Check sheet for the modelled part. Datum: model origin and axes. Units: mm. Coordinates: 2 decimals unless noted, no trailing zeros. Write each loop counter-clockwise with the first axis right and the second up, starting at its lowest first coordinate (ties: lowest second). Pieces come first, ordered by that corner, then holes. Notation, with made-up numbers: (60, -10) -> (74, -10) arc R20 cw to (74, 6) -> close; hole circle Ø2 at (-14.75, 35). An arc over 180 degrees is marked (long way). One line per item, written item: value. Start each with the question number.
1) Sectioned sample at C-C on z = -468.5. Enter the section's corners in (x, y) (3 decimals).
2) Scan lines: line 1 along Z through (x, y) = (0.95, 40.5); line 2 along Z through (x, y) = (2.95, 4.5); line 3 along Z through (x, y) = (0.9, 41). Record each from-to range of solid material in increasing order. Write a range as [from, to].
3) Sectioned sample at A-A on z = -557.53. Enter the section's corners in (x, y) (3 decimals), plus the area to 3 significant figures.
4) Gauge pin test, flat ends, axial feed: P1, Ø5.5, axis at y = 15.875, z = -431.8, coming from the +X side; P2, Ø1.6, axis at x = 1, z = -849, coming from the +Y side; P3, Ø1.5, axis at x = 2, z = -437, coming from the -Y side (3 decimals); P4, Ø1, axis at x = 1.5, y = 59, coming from the +Z side. Record the tip position at first contact, or that the pin passes through.
5) Sectioned sample at B-B on x = 2.6. Give the number of separate pieces and of enclosed holes in the cut face, plus the area to 3 significant figures.
Autodesk Inventor part; units mm, degrees
ref_plane "YZ Plane" through (0, 0, 0) normal (1, 0, 0) x (0, 1, 0)
ref_plane "XZ Plane" through (0, 0, 0) normal (0, 1, 0) x (-1, 0, 0)
ref_plane "XY Plane" through (0, 0, 0) normal (0, 0, 1) x (1, 0, 0)
sketch "Sketch1" plane through (0, 0, 0) normal (1, 0, 0) x (0, 1, 0)
  line L0 (0, 0) -> (76.2, 0)
  line L1 (76.2, 0) -> (76.2, -863.6)
  line L2 (76.2, -863.6) -> (0, -863.6)
  line L3 (0, -863.6) -> (0, 0)
  dimension "d0" = 76.2
  dimension "d1" = 863.6
extrude "Extrusion1" add sketch "Sketch1" along normal blind 3.175
sketch "Sketch2" plane through (3.175, 0, 0) normal (1, 0, 0) x (0, 0, -1)
  line L0 (0, 38.1) -> (0, 36.5125)
  line L1 (0, 36.5125) -> (0, 39.6875)
  circle A0 centre (306.07, 36.5125) radius 14.2875
  circle A1 centre (557.53, 36.5125) radius 14.2875
  circle A2 centre (105.4351, 39.6875) radius 14.2875
  circle A3 centre (758.1649, 39.6875) radius 14.2875
  line L2 (863.6, 0) -> (838.2, 0)
  line L3 (863.6, 0) -> (863.6, 38.1)
  line L4 (863.6, 38.1) -> (838.2, 0)
  circle A4 centre (12.7, 63.5) radius 3.175
  line L5 (863.6, 76.2) -> (0, 76.2)
  circle A5 centre (850.9, 63.5) radius 3.175
  circle A6 centre (825.5, 15.875) radius 3.175
  circle A7 centre (38.1, 15.875) radius 3.175
  circle A8 centre (190.5, 15.875) radius 3.175
  circle A9 centre (431.8, 15.875) radius 3.175
  circle A10 centre (431.8, 63.5) radius 3.175
  circle A11 centre (673.1, 63.5) radius 3.175
  circle A12 centre (673.1, 15.875) radius 3.175
  circle A13 centre (190.5, 63.5) radius 3.175
  line L6 (0, 0) -> (25.4, 0)
  line L7 (0, 0) -> (0, 38.1)
  line L8 (0, 38.1) -> (25.4, 0)
  line L9 (863.6, 0) -> (0, 0)
  dimension "d15" = 28.575
  dimension "d16" = 28.575
  dimension "d19" = 28.575
  dimension "d21" = 28.575
  dimension "d22" = 25.4
  dimension "d26" = 6.35
  dimension "d27" = 12.7
  dimension "d29" = 6.35
  dimension "d30" = 12.7
  dimension "d32" = 6.35
  dimension "d34" = 12.7
  dimension "d35" = 6.35
  dimension "d39" = 6.35
  dimension "d40" = 863.6
  dimension "d41" = 6.35
  dimension "d43" = 6.35
  dimension "d44" = 12.7
  dimension "d45" = 6.35
  dimension "d46" = 6.35
  dimension "d48" = 241.3
  dimension "d49" = 241.3
  dimension "d50" = 6.35
  dimension "d51" = 241.3
  dimension "d53" = 241.3
  dimension "d54" = 25.4
  dimension "d55" = 38.1
  dimension "d58" = 15.875
  dimension "d59" = 15.875
  dimension "d60" = 15.875
extrude "Extrusion3" cut sketch "Sketch2" against normal blind 25.4
sketch "Sketch3" plane through (3.175, 0, 0) normal (1, 0, 0) x (0, 0, -1)
  line L0 (0, 76.2) -> (863.6, 76.2)
  line L1 (0, 76.2) -> (25.4, 76.2)
  line L2 (25.4, 76.2) -> (25.4, 50.8)
  line L3 (25.4, 50.8) -> (0, 50.8)
  line L4 (0, 50.8) -> (0, 76.2)
  line L5 (25.4, 0) -> (50.8, 0)
  line L6 (50.8, 0) -> (50.8, 28.575)
  line L7 (50.8, 28.575) -> (25.4, 28.575)
  line L8 (25.4, 28.575) -> (25.4, 0)
  line L9 (863.6, 76.2) -> (838.2, 76.2)
  line L10 (838.2, 76.2) -> (838.2, 50.8)
  line L11 (838.2, 50.8) -> (863.6, 50.8)
  line L12 (863.6, 50.8) -> (863.6, 76.2)
  line L13 (50.8, 0) -> (812.8, 0)
  line L14 (812.8, 0) -> (812.8, 3.175)
  line L15 (812.8, 3.175) -> (50.8, 3.175)
  line L16 (50.8, 3.175) -> (50.8, 0)
  line L17 (838.2, 0) -> (812.8, 0)
  line L18 (812.8, 0) -> (812.8, 28.575)
  line L19 (812.8, 28.575) -> (838.2, 28.575)
  line L20 (838.2, 28.575) -> (838.2, 0)
  circle A0 centre (38.1, 63.5) radius 3.175
  circle A1 centre (825.5, 63.5) radius 3.175
  circle A2 centre (306.07, 36.5125) radius 14.2875
  circle A3 centre (329.8825, 36.5125) radius 2.413
  circle A4 centre (363.22, 36.5125) radius 2.413
  circle A5 centre (282.2575, 36.5125) radius 2.413
  circle A6 centre (248.92, 36.5125) radius 2.413
  point P0 (0, 0)
  dimension "d63" = 25.4
  dimension "d64" = 25.4
  dimension "d65" = 25.4
  dimension "d66" = 28.575
  dimension "d67" = 25.4
  dimension "d68" = 25.4
  dimension "d77" = 762
  dimension "d78" = 3.175
  dimension "d79" = 25.4
  dimension "d80" = 28.575
  dimension "d81" = 6.35
  dimension "d82" = 6.35
  dimension "d88" = 4.826
  dimension "d89" = 4.826
  dimension "d90" = 4.826
  dimension "d91" = 4.826
extrude "Extrusion5" cut sketch "Sketch3" against normal blind 25.4 contours L0 L12 L11 L10 | L0 L2 L3 L4 | L8 L7 L6 L5 | L6 L15 L14 L13 | L14 L18 L19 L20 L17 | A0 | A1 | A3 | A4 | A5 | A6
properties part number "InsidePlate"
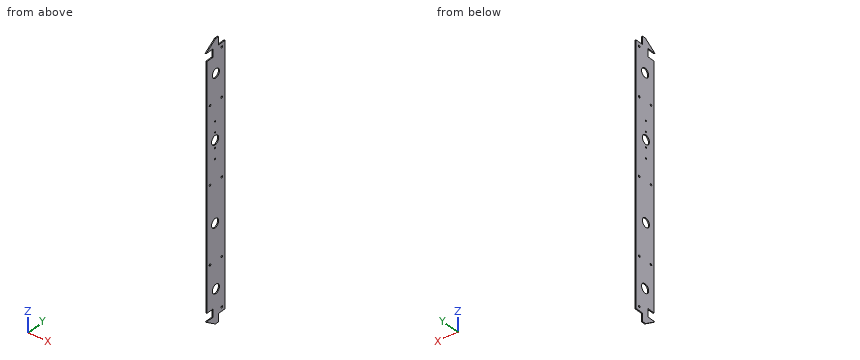
Answers:
1. outline: (0, 3.175) -> (3.175, 3.175) -> (3.175, 76.2) -> (0, 76.2) -> close
2. line 1: z = [-863.6, -772.43], [-743.9, -571.25], [-543.81, -319.79], [-292.35, -119.7], [-91.17, 0]
2. line 2: z = [-841.2, -838.2], [-812.8, -50.8], [-25.4, -22.4]
2. line 3: z = [-863.6, -772.39], [-743.94, -571.09], [-543.97, -319.63], [-292.51, -119.66], [-91.21, 0]
3. outline: (0, 3.175) -> (3.175, 3.175) -> (3.175, 22.225) -> (0, 22.225) -> close; (0, 50.8) -> (3.175, 50.8) -> (3.175, 76.2) -> (0, 76.2) -> close
3. area: 141 mm2
4. P1: passes through
4. P2: stops at y = 50.8
4. P3: stops at y = 3.175
4. P4: stops at z = -25.4
5. separate pieces: 1
5. enclosed holes: 16
5. area: 56,800 mm2
